Check sheet for the modelled part. Datum: model origin and axes. Units: mm. A direction names the side the tool comes from. Give positions to 0.01 mm unless a question says otherwise; leave off trailing zeros. Order: outer loops, then holes, each group sorted by start corner. A loop starts at its lowest first (then second) coordinate and runs counter-clockwise, first axis right, second up. Notation, with made-up numbers: (12.5, -27) -> (31.5, -27) arc R18 cw to (31.5, -7) -> close; hole circle Ø10 at (87, 53). An arc over 180 degrees is marked (long way). Write each question's results on one line, items separated by ' | '.
from build123d import *

# Parameters (mm, degrees)
BOSS_EXTRUDE1_DEPTH      = 1
SKETCH2_R                = 1.325
CUT_EXTRUDE1_DEPTH       = 36.80851854
SKETCH3_R                = 0.5
CUT_EXTRUDE2_DEPTH       = 36.80851854
LPATTERN1_COUNT          = 20
LPATTERN1_PITCH          = 2.54
BOSS_EXTRUDE6_DEPTH      = 1.25
BOSS_EXTRUDE6_DEPTH_BACK = 4.5
CUT_EXTRUDE9_DEPTH       = 5.25
SKETCH_1_W               = 4.7
SKETCH_1_H               = 2.3
EXTRUDE_1_DEPTH          = 2
SKETCH_2_W               = 1.86
SKETCH_2_H               = 1
EXTRUDE_2_DEPTH          = 1
SKETCH_9_R               = 2.75
SKETCH_9_R_2             = 1.325
EXTRUDE_8_DEPTH          = 1.5
SKETCH_10_R              = 1.05
EXTRUDE_9_DEPTH          = 2.5
SKETCH_11_R              = 0.5
EXTRUDE_10_DEPTH         = 3
SKETCH_12_R              = 7
EXTRUDE_11_DEPTH         = 2


with BuildPart() as part:
    # Sketch1 → Boss-Extrude1 (new body)
    with BuildSketch(Plane(origin=(0, 0, 0), x_dir=(1, 0, 0), z_dir=(0, 1, 0))):
        with BuildLine():
            Line((-28.75, 15), (28.75, 15))
            ThreePointArc((28.75, 15), (31.401650429, 13.901650429), (32.5, 11.25))
            Line((32.5, 11.25), (32.5, -11.25))
            ThreePointArc((32.5, -11.25), (31.401650429, -13.901650429), (28.75, -15))
            Line((28.75, -15), (-28.75, -15))
            ThreePointArc((-28.75, -15), (-31.401650429, -13.901650429), (-32.5, -11.25))
            Line((-32.5, -11.25), (-32.5, 11.25))
            ThreePointArc((-32.5, 11.25), (-31.401650429, 13.901650429), (-28.75, 15))
        make_face()
    extrude(amount=BOSS_EXTRUDE1_DEPTH)

    # Sketch2 → Cut-Extrude1 (cut, through all)
    with BuildSketch(Plane(origin=(0, 1, 0), x_dir=(1, 0, 0), z_dir=(0, 1, 0))):
        with Locations(Location((-29.025, 11.525, 0), (0, 0, 270))):
            Circle(SKETCH2_R)
        with Locations(Location((29.025, 11.525, 0), (0, 0, 90))):
            Circle(SKETCH2_R)
        with Locations(Location((29.025, -11.525, 0), (0, 0, 270))):
            Circle(SKETCH2_R)
        with Locations(Location((-29.025, -11.525, 0), (0, 0, 90))):
            Circle(SKETCH2_R)
    extrude(amount=-CUT_EXTRUDE1_DEPTH, mode=Mode.SUBTRACT)

    # Sketch3 → Cut-Extrude2 (cut, through all)
    with BuildSketch(Plane(origin=(0, 1, 0), x_dir=(1, 0, 0), z_dir=(0, 1, 0))):
        with Locations(Location((-24.128, 13, 0), (0, 0, 270))):
            Circle(SKETCH3_R)
        with Locations(Location((-24.128, 10.5, 0), (0, 0, 270))):
            Circle(SKETCH3_R)
    cut_extrude2 = extrude(amount=-CUT_EXTRUDE2_DEPTH, mode=Mode.SUBTRACT)

    # LPattern1: Cut-Extrude2 ×20
    with Locations(*[(i * LPATTERN1_PITCH, 0, 0) for i in range(1, LPATTERN1_COUNT)]):
        add(cut_extrude2, mode=Mode.SUBTRACT)

    # Sketch15 → Boss-Extrude6 (add, two sides: drawn at the far end of the back side and taken through both)
    with BuildSketch(Plane.XY.offset(15).offset(-BOSS_EXTRUDE6_DEPTH_BACK)):
        with BuildLine():
            Line((-24, 4), (-17, 4))
            ThreePointArc((-17, 4), (-16.292893219, 3.707106781), (-16, 3))
            Line((-16, 3), (-16, 2))
            ThreePointArc((-16, 2), (-16.292893219, 1.292893219), (-17, 1))
            Line((-17, 1), (-24, 1))
            ThreePointArc((-24, 1), (-24.707106781, 1.292893219), (-25, 2))
            Line((-25, 2), (-25, 3))
            ThreePointArc((-25, 3), (-24.707106781, 3.707106781), (-24, 4))
        make_face()
    extrude(amount=BOSS_EXTRUDE6_DEPTH + BOSS_EXTRUDE6_DEPTH_BACK)

    # Sketch16 → Cut-Extrude9 (cut)
    with BuildSketch(Plane.XY.offset(16.25)):
        with BuildLine():
            Line((-17, 3.68), (-24, 3.68))
            ThreePointArc((-24, 3.68), (-24.480832611, 3.480832611), (-24.68, 3))
            Line((-24.68, 3), (-24.68, 2))
            ThreePointArc((-24.68, 2), (-24.480832611, 1.519167389), (-24, 1.32))
            Line((-24, 1.32), (-17, 1.32))
            ThreePointArc((-17, 1.32), (-16.519167389, 1.519167389), (-16.32, 2))
            Line((-16.32, 2), (-16.32, 3))
            ThreePointArc((-16.32, 3), (-16.519167389, 3.480832611), (-17, 3.68))
        make_face()
    extrude(amount=-CUT_EXTRUDE9_DEPTH, mode=Mode.SUBTRACT)

    # 草图1 → 凸台-拉伸1 (add)
    with BuildSketch(Plane(origin=(0, 1, 0), x_dir=(1, 0, 0), z_dir=(0, 1, 0))):
        with Locations((-10.52, -13.05)):
            Rectangle(SKETCH_1_W, SKETCH_1_H)
        with Locations((21.95, -13.05)):
            Rectangle(SKETCH_1_W, SKETCH_1_H)
    extrude(amount=EXTRUDE_1_DEPTH)

    # 草图2 → 凸台-拉伸2 (add)
    with BuildSketch(Plane.XY.offset(14.2)):
        with Locations((-10.52, 2)):
            Rectangle(SKETCH_2_W, SKETCH_2_H)
        with Locations((21.95, 2)):
            Rectangle(SKETCH_2_W, SKETCH_2_H)
    extrude(amount=EXTRUDE_2_DEPTH)

    # 草图9 → 凸台-拉伸8 (add)
    # profile 1 of 4: a face of its own
    with BuildSketch(Plane.XZ):
        with Locations(Location((29.025, 11.525, 0), (0, 0, 90))):
            Circle(SKETCH_9_R)
        with Locations(Location((29.025, 11.525, 0), (0, 0, 90))):
            Circle(SKETCH_9_R_2, mode=Mode.SUBTRACT)
    # profile 2 of 4: a face of its own
    with BuildSketch(Plane.XZ):
        with Locations(Location((29.025, -11.525, 0), (0, 0, 90))):
            Circle(SKETCH_9_R)
        with Locations(Location((29.025, -11.525, 0), (0, 0, 270))):
            Circle(SKETCH_9_R_2, mode=Mode.SUBTRACT)
    # profile 3 of 4: a face of its own
    with BuildSketch(Plane.XZ):
        with Locations(Location((-29.025, 11.525, 0), (0, 0, 90))):
            Circle(SKETCH_9_R)
        with Locations(Location((-29.025, 11.525, 0), (0, 0, 270))):
            Circle(SKETCH_9_R_2, mode=Mode.SUBTRACT)
    # profile 4 of 4: a face of its own
    with BuildSketch(Plane.XZ):
        with Locations(Location((-29.025, -11.525, 0), (0, 0, 90))):
            Circle(SKETCH_9_R)
        with Locations(Location((-29.025, -11.525, 0), (0, 0, 90))):
            Circle(SKETCH_9_R_2, mode=Mode.SUBTRACT)
    extrude(amount=EXTRUDE_8_DEPTH)

    # 草图10 → 凸台-拉伸9 (add)
    with BuildSketch(Plane(origin=(0, 1, 0), x_dir=(1, 0, 0), z_dir=(0, 1, 0))):
        with Locations(Location((24.132, 13, 0), (0, 0, 270))):
            Circle(SKETCH_10_R)
        with Locations(Location((21.592, 13, 0), (0, 0, 270))):
            Circle(SKETCH_10_R)
        with Locations(Location((19.052, 13, 0), (0, 0, 270))):
            Circle(SKETCH_10_R)
        with Locations(Location((21.592, 10.5, 0), (0, 0, 270))):
            Circle(SKETCH_10_R)
        with Locations(Location((19.052, 10.5, 0), (0, 0, 270))):
            Circle(SKETCH_10_R)
        with Locations(Location((-24.128, 10.5, 0), (0, 0, 270))):
            Circle(SKETCH_10_R)
    extrude(amount=EXTRUDE_9_DEPTH)

    # 草图11 → 凸台-拉伸10 (add)
    with BuildSketch(Plane.XZ.offset(-1)):
        with Locations(Location((24.132, -13, 0), (0, 0, 90))):
            Circle(SKETCH_11_R)
        with Locations(Location((21.592, -13, 0), (0, 0, 90))):
            Circle(SKETCH_11_R)
        with Locations(Location((21.592, -10.5, 0), (0, 0, 90))):
            Circle(SKETCH_11_R)
        with Locations(Location((19.052, -10.5, 0), (0, 0, 90))):
            Circle(SKETCH_11_R)
        with Locations(Location((19.052, -13, 0), (0, 0, 90))):
            Circle(SKETCH_11_R)
        with Locations(Location((-24.128, -10.5, 0), (0, 0, 90))):
            Circle(SKETCH_11_R)
    extrude(amount=EXTRUDE_10_DEPTH)

    # 草图12 → 凸台-拉伸11 (add)
    with BuildSketch(Plane(origin=(0, 1, 0), x_dir=(1, 0, 0), z_dir=(0, 1, 0))):
        with Locations(Location((12.5, 0, 0), (0, 0, 270))):
            Circle(SKETCH_12_R)
    extrude(amount=EXTRUDE_11_DEPTH)


solid = part.part
1. Mould release check, pull along X, two halves, no side actions. Record for faces 6 (the cylindrical face through (31.431, 0.493, 13.872)), 7 (the flat face through (0, 0, 0)), 8 (the flat face through (-24, 3.5, -11)), 9 (the cylindrical face through (18.12, 2.23, -10.02)): +X half, -X half, draft (parallel to the pull), parting line (faces both ways), or undercut.
Verdict:
face 6: +X half | face 7: undercut | face 8: draft | face 9: undercut
2. Gauge pin test, flat ends, axial feed: pin 1 Ø1 at (x, z) = (-18.5, -10.5) entering from +Y; pin 2 Ø4 at (x, z) = (-29.025, -11.525) entering from -Y; pin 3 Ø0.5 at (x, y) = (22, 2) entering from +Z. Record the tip position at first contact, or that the pin passes through.
Verdict:
pin 1: stops at y = 1 | pin 2: stops at y = -1.5 | pin 3: stops at z = 15.2
3. Section check B-B on x = 10. Record the cut outline in (y, z), then the cut area to 3 significant figures.
Verdict:
outline: (0, -15) -> (1, -15) -> (1, -6.54) -> (3, -6.54) -> (3, 6.54) -> (1, 6.54) -> (1, 15) -> (0, 15) -> close | area: 56.2 mm^2
4. Access from +Z, -Z, +X, -X, +Y, -Y to the whole of each face (thin tool, end or side, straight path). Record for faces 1 (the flat face through (28, -1.5, -10)), 2 (the flat face through (-30, -1.5, -10)), 3 (the flat face through (24.3, 2, 13)), 4 (the flat face through (-20, 1, 16)), 5 (the cylindrical face through (22.633, 2.232, -13.137)).
Verdict:
face 1: +Z, -Z, +X, -Y | face 2: +Z, -Z, -X, -Y | face 3: +Z, +X, +Y | face 4: +Z, +X, -X, -Y | face 5: +Y
5. Section check A-A on z = -0.5. Record the cut outline in (x, y).
Verdict:
outline: (-32.5, 0) -> (32.5, 0) -> (32.5, 1) -> (19.48, 1) -> (19.48, 3) -> (5.52, 3) -> (5.52, 1) -> (-32.5, 1) -> close
6. Material ranges on probe 1 along Z at (x, y) = (9, 0.5); probe 2 along Y at (x, z) = (-19, 13); probe 3 along X at (y, z) = (3.15, -11), recorded low to high. Write a range as from..to.
Verdict:
probe 1: z = -15..-13.49, -12.51..-10.99, -10.01..15 | probe 2: y = 0..1.32, 3.68..4 | probe 3: x = -25.05..-23.2, 18.13..19.98, 20.67..22.52
